Verification items for the finished model (mm, model axes). A direction names the side the tool comes from. Coordinates: 2 decimals unless noted, no trailing zeros. Write item = value, one per line.
```python
from build123d import *

# Parameters (mm, degrees)
ESQUISSE1_R             = 56.5
BOSS_EXTRU_1_DEPTH      = 24
ESQUISSE1_R_2           = 26
BOSS_EXTRU_1_2_DEPTH    = 24
ENL_V_MAT_EXTRU_1_DEPTH = 172.394282285
CONG_1_R                = 0.5
CONG_2_R                = 2
BOSS_EXTRU_2_START      = -5
BOSS_EXTRU_2_DEPTH      = 5
CONG_3_R                = 2
ESQUISSE4_R             = 2.25
ENL_V_MAT_EXTRU_2_DEPTH = 172.394282299


# Some blends are built 0.0001 mm under size
with BuildPart() as part:
    # Esquisse1 → Boss.-Extru.1 (new body)
    with BuildSketch(Plane.XY):
        Polygon((0, 95), (0, 0), (120, 0), (120, 120), (32.113356809, 120), (0.4, 120), (0, 120), (0, 114.342406945), align=None)
        with Locations((60, 60)):
            Circle(ESQUISSE1_R, mode=Mode.SUBTRACT)
    extrude(amount=BOSS_EXTRU_1_DEPTH)

    # Esquisse2 → Enlèv. mat.-Extru.1 (cut, through all)
    with BuildSketch(Plane.XY.offset(24)):
        Polygon((0, 94), (0.5, 94), (0.5, 119.5), (26, 119.5), (26, 120), (0, 120), align=None)
        Polygon((26, 0.5), (26, 0), (0, 0), (0, 26), (0.5, 26), (0.5, 0.5), align=None)
        Polygon((120, 0), (94, 0), (94, 0.5), (119.5, 0.5), (119.5, 26), (120, 26), align=None)
        Polygon((120, 120), (94, 120), (94, 119.5), (119.5, 119.5), (119.5, 94), (120, 94), align=None)
    extrude(amount=-ENL_V_MAT_EXTRU_1_DEPTH, mode=Mode.SUBTRACT)

    # Congé1
    cong_1_edges = [part.edges().sort_by_distance(p)[0] for p in [
        (94, 119.5, 12),
        (119.5, 94, 12),
        (94, 0.5, 12),
        (119.5, 26, 12),
        (26, 0.5, 12),
        (0.5, 26, 12),
        (0.5, 94, 12),
        (26, 119.5, 12),
    ]]
    fillet(cong_1_edges, radius=CONG_1_R - 0.0001)  # a hair under: the kernel refuses the full size

    # Congé2
    cong_2_edges = [part.edges().sort_by_distance(p)[0] for p in [
        (119.5, 119.5, 12),
        (119.5, 0.5, 12),
        (0.5, 0.5, 12),
        (0.5, 119.5, 12),
    ]]
    fillet(cong_2_edges, radius=CONG_2_R)



with BuildPart() as body_2:
    # Esquisse1 → Boss.-Extru.1 2 (new body)
    with BuildSketch(Plane.XY):
        with Locations((60, 60)):
            Circle(ESQUISSE1_R_2)
    extrude(amount=BOSS_EXTRU_1_2_DEPTH)


with BuildPart() as part_1:
    add(part.part)

    add(body_2.part)  # Boss.-Extru.2 merges body 2
    # Esquisse3 → Boss.-Extru.2 (add)
    with BuildSketch(Plane.XY.offset(24).offset(BOSS_EXTRU_2_START)):
        with BuildLine():
            ThreePointArc((3.724458924, 65.03125), (3.506910291, 60.883637464), (3.594634356, 56.73125))
            ThreePointArc((3.594634356, 56.73125), (20.845057368, 69.763102479), (40.955053164, 77.7))
            ThreePointArc((40.955053164, 77.7), (49.612507521, 83.834848437), (60, 86))
            ThreePointArc((60, 86), (29.972408521, 80.587491275), (3.724458924, 65.03125))
        make_face()
        with BuildLine():
            ThreePointArc((65.03125, 116.275541076), (60.883637464, 116.493089709), (56.73125, 116.405365644))
            ThreePointArc((56.73125, 116.405365644), (69.763102479, 99.154942632), (77.7, 79.044946836))
            ThreePointArc((77.7, 79.044946836), (83.834848437, 70.387492479), (86, 60))
            ThreePointArc((86, 60), (80.587491275, 90.027591479), (65.03125, 116.275541076))
        make_face()
        with BuildLine():
            ThreePointArc((60, 34), (90.027591479, 39.412508725), (116.275541076, 54.96875))
            ThreePointArc((116.275541076, 54.96875), (116.443857375, 57.481872801), (116.5, 60))
            ThreePointArc((116.5, 60), (116.476336456, 61.635059802), (116.405365644, 63.26875))
            ThreePointArc((116.405365644, 63.26875), (99.154942632, 50.236897521), (79.044946836, 42.3))
            ThreePointArc((79.044946836, 42.3), (70.387492479, 36.165151563), (60, 34))
        make_face()
        with BuildLine():
            ThreePointArc((34, 60), (39.412508725, 29.972408521), (54.96875, 3.724458924))
            ThreePointArc((54.96875, 3.724458924), (59.116362536, 3.506910291), (63.26875, 3.594634356))
            ThreePointArc((63.26875, 3.594634356), (50.236897521, 20.845057368), (42.3, 40.955053164))
            ThreePointArc((42.3, 40.955053164), (36.165151563, 49.612507521), (34, 60))
        make_face()
    extrude(amount=BOSS_EXTRU_2_DEPTH)

    # Congé3
    # the kernel refuses this fillet: 2 mm, written as the material it takes off along each edge
    with BuildSketch(Plane(origin=(60, 0, 19), x_dir=(0.17354982017034465, 0.9848250910282704, 0), z_dir=(0.9848250910282704, -0.17354982017034465, 0))) as cong_3_piece_1_section:
        with BuildLine():
            CenterArc((86 - CONG_3_R, CONG_3_R), CONG_3_R, 270, 90)
            Line((86, CONG_3_R), (86, 0))
            Line((86, 0), (86 - CONG_3_R, 0))
        make_face()
    cong_3_piece_1 = revolve(axis=Axis((60, 0, 19), (0, 0, 1)), revolution_arc=54.197355046, mode=Mode.PRIVATE)
    cong_3_piece_1 = cong_3_piece_1 & Plane(origin=(60, 60, 19), x_dir=(1, 0, 0), z_dir=(0, 0, -1)) * Cylinder(56.5, 344, mode=Mode.PRIVATE)
    cong_3_piece_1 = cong_3_piece_1 - Plane(origin=(60, 60, 19), x_dir=(1, 0, 0), z_dir=(0, 0, -1)) * Cylinder(26, 344, mode=Mode.PRIVATE)
    add(cong_3_piece_1, mode=Mode.SUBTRACT)
    with BuildSketch(Plane(origin=(0, 60, 19), x_dir=(0.9848250910282706, -0.17354982017034323, 0), z_dir=(-0.17354982017034323, -0.9848250910282706, 0))) as cong_3_piece_2_section:
        with BuildLine():
            CenterArc((86 - CONG_3_R, CONG_3_R), CONG_3_R, 270, 90)
            Line((86, CONG_3_R), (86, 0))
            Line((86, 0), (86 - CONG_3_R, 0))
        make_face()
    cong_3_piece_2 = revolve(axis=Axis((0, 60, 19), (0, 0, 1)), revolution_arc=54.197355046, mode=Mode.PRIVATE)
    cong_3_piece_2 = cong_3_piece_2 & Plane(origin=(60, 60, 19), x_dir=(1, 0, 0), z_dir=(0, 0, -1)) * Cylinder(56.5, 345, mode=Mode.PRIVATE)
    cong_3_piece_2 = cong_3_piece_2 - Plane(origin=(60, 60, 19), x_dir=(1, 0, 0), z_dir=(0, 0, -1)) * Cylinder(26, 345, mode=Mode.PRIVATE)
    add(cong_3_piece_2, mode=Mode.SUBTRACT)
    with BuildSketch(Plane(origin=(60, 120, 19), x_dir=(-0.17354982017035084, -0.9848250910282692, 0), z_dir=(-0.9848250910282692, 0.17354982017035084, 0))) as cong_3_piece_3_section:
        with BuildLine():
            CenterArc((86 - CONG_3_R, CONG_3_R), CONG_3_R, 270, 90)
            Line((86, CONG_3_R), (86, 0))
            Line((86, 0), (86 - CONG_3_R, 0))
        make_face()
    cong_3_piece_3 = revolve(axis=Axis((60, 120, 19), (0, 0, 1)), revolution_arc=54.197355046, mode=Mode.PRIVATE)
    cong_3_piece_3 = cong_3_piece_3 & Plane(origin=(60, 60, 19), x_dir=(1, 0, 0), z_dir=(0, 0, -1)) * Cylinder(56.5, 344, mode=Mode.PRIVATE)
    cong_3_piece_3 = cong_3_piece_3 - Plane(origin=(60, 60, 19), x_dir=(1, 0, 0), z_dir=(0, 0, -1)) * Cylinder(26, 344, mode=Mode.PRIVATE)
    add(cong_3_piece_3, mode=Mode.SUBTRACT)
    with BuildSketch(Plane(origin=(120, 60, 19), x_dir=(-0.9848250910282709, 0.17354982017034223, 0), z_dir=(0.17354982017034223, 0.9848250910282709, 0))) as cong_3_piece_4_section:
        with BuildLine():
            CenterArc((86 - CONG_3_R, CONG_3_R), CONG_3_R, 270, 90)
            Line((86, CONG_3_R), (86, 0))
            Line((86, 0), (86 - CONG_3_R, 0))
        make_face()
    cong_3_piece_4 = revolve(axis=Axis((120, 60, 19), (0, 0, 1)), revolution_arc=54.197355046, mode=Mode.PRIVATE)
    cong_3_piece_4 = cong_3_piece_4 & Plane(origin=(60, 60, 19), x_dir=(1, 0, 0), z_dir=(0, 0, -1)) * Cylinder(56.5, 344, mode=Mode.PRIVATE)
    cong_3_piece_4 = cong_3_piece_4 - Plane(origin=(60, 60, 19), x_dir=(1, 0, 0), z_dir=(0, 0, -1)) * Cylinder(26, 344, mode=Mode.PRIVATE)
    add(cong_3_piece_4, mode=Mode.SUBTRACT)

    # Esquisse4 → Enlèv. mat.-Extru.2 (cut, through all)
    with BuildSketch(Plane(origin=(0, 0, 0), x_dir=(-1, 0, 0), z_dir=(0, 0, -1))):
        with Locations((-7.5, 112.5)):
            Circle(ESQUISSE4_R)
        with Locations(Location((-112.5, 112.5, 0), (0, 0, 180))):
            Circle(ESQUISSE4_R)
        with Locations(Location((-7.5, 7.5, 0), (0, 0, 180))):
            Circle(ESQUISSE4_R)
        with Locations((-112.5, 7.5)):
            Circle(ESQUISSE4_R)
    extrude(amount=-ENL_V_MAT_EXTRU_2_DEPTH, mode=Mode.SUBTRACT)


solid = part_1.part
```
Item 1: Gauge pin test, flat ends, axial feed: pin 1 (4 mm diameter, centred on x = 79, z = 20, fed in from -Y); pin 2 (5 mm diameter, centred on x = 104, z = 17.5, fed in from -Y); pin 3 (21 mm diameter, centred on x = 73, y = 96, fed in from -Z); pin 4 (11.5 mm diameter, centred on y = 10, z = 10, fed in from +X). Record the tip position at first contact, or that the pin passes through.
Report:
pin_1 = 0
pin_2 = 0.5
pin_3 = 19
pin_4 = 119.5
Item 2: Scan lines: L1, parallel to Y at x = 60, z = 5; L2, parallel to Y at x = 82, z = 5.25; L3, parallel to Y at x = 8, z = 13.75. Record each from-to range of solid material in increasing order. Write a range as from..to.
Report:
L1 = 0..3.5, 34..86, 116.5..120
L2 = 0..7.96, 46.14..73.86, 112.04..120
L3 = 0.5..5.31, 9.69..37.9, 82.1..110.31, 114.69..119.5
Item 3: Sectioned sample at A-A, the plane z = 17.5. Give the number of separate pieces and of enclosed holes in the cut face, then the cut area to 3 significant figures.
Report:
separate_pieces = 2
enclosed_holes = 5
area = 6,330 mm^2
Item 4: Tool access check on faces 4 (the flat face through (119.5, 106, 12)), 5 (the flat face through (22, 71, 19)), 6 (the flat face through (120, 60, 12)), 7 (the flat face through (14, 119.5, 12)), 8 (the cylindrical face through (7.988, 110.304, 11.832)). Record the directions out of +Z, -Z, +X, -X, +Y, -Y that give a thin tool (end or side, any length) a straight path to the whole face; none if there is none.
Report:
face_4 = +Z, -Z, +X, +Y
face_5 = -Z
face_6 = +Z, -Z, +X, +Y, -Y
face_7 = +Z, -Z, -X, +Y
face_8 = +Z, -Z
Item 5: Release check for a two-part mould opening along X. For faces 1 (the flat face through (59, 61, 24)), 2 (the flat face through (119.5, 14, 12)), 3 (the flat face through (48, 23, 19)) record: pulls with the +X half, pulls with the -X half, needs draft (parallel to the pull), parting line crosses it, or undercut.
Report:
face_1 = needs draft
face_2 = pulls with the +X half
face_3 = undercut
